```python
from build123d import *

# Parameters (mm, degrees)
ESQUISSE1_R        = 5.5
BOSS_EXTRU_1_DEPTH = 5
ESQUISSE2_W        = 33
ESQUISSE2_H        = 10
ESQUISSE2_W_2      = 10
ESQUISSE2_H_2      = 24.25
ESQUISSE2_H_3      = 12.75
BOSS_EXTRU_2_DEPTH = 6
D_POUILLE1_ANGLE   = 10
BOSS_EXTRU_3_DEPTH = 10
CHANFREIN1_SIZE    = 5


with BuildPart() as part:
    # Esquisse1 → Boss.-Extru.1 (new body)
    with BuildSketch(Plane.XY):
        Polygon((-22.5, 75.232443508), (22.5, 75.232443508), (70, -9.767556492), (70, -54.767556492), (-70, -54.767556492), (-70, -9.767556492), align=None)
        with Locations((0, 60.232443508)):
            Circle(ESQUISSE1_R, mode=Mode.SUBTRACT)
        with Locations((0, 13.982443508)):
            Circle(ESQUISSE1_R, mode=Mode.SUBTRACT)
        with Locations((0, -32.267556492)):
            Circle(ESQUISSE1_R, mode=Mode.SUBTRACT)
        with Locations((-55, -32.267556492)):
            Circle(ESQUISSE1_R, mode=Mode.SUBTRACT)
        with Locations((55, -32.267556492)):
            Circle(ESQUISSE1_R, mode=Mode.SUBTRACT)
    extrude(amount=BOSS_EXTRU_1_DEPTH)

    # Esquisse2 → Boss.-Extru.2 (add)
    with BuildSketch(Plane.XY.offset(5)):
        with Locations((-27.5, -32.267556492)):
            Rectangle(ESQUISSE2_W, ESQUISSE2_H)
        with Locations((27.5, -32.267556492)):
            Rectangle(ESQUISSE2_W, ESQUISSE2_H)
        with Locations((0, 37.107443508)):
            Rectangle(ESQUISSE2_W_2, ESQUISSE2_H_2)
        with Locations((0, -3.392556492)):
            Rectangle(ESQUISSE2_W_2, ESQUISSE2_H_3)
    extrude(amount=BOSS_EXTRU_2_DEPTH)

    # Dépouille1
    d_pouille1_faces = [part.faces().sort_by_distance(p)[0] for p in [
        (44, -32.267556492, 8),
        (27.5, -27.267556492, 8),
        (-11, -32.267556492, 8),
        (-27.5, -27.267556492, 8),
        (0, 2.982443508, 8),
        (5, -3.392556492, 8),
        (0, 49.232443508, 8),
        (5, 37.107443508, 8),
        (-5, 37.107443508, 8),
        (0, 24.982443508, 8),
        (11, -32.267556492, 8),
        (-44, -32.267556492, 8),
        (-5, -3.392556492, 8),
        (-27.5, -37.267556492, 8),
        (27.5, -37.267556492, 8),
        (0, -9.767556492, 8),
    ]]
    draft(d_pouille1_faces, Plane.XY.offset(5), D_POUILLE1_ANGLE)

    # Esquisse3 → Boss.-Extru.3 (add)
    with BuildSketch(Plane.XY.offset(5)):
        Polygon((-22.75, 74.785075087), (-22.75, -9.517556492), (-69.860294118, -9.517556492), align=None)
        Polygon((22.75, -9.517556492), (69.860294118, -9.517556492), (22.75, 74.785075087), align=None)
    extrude(amount=BOSS_EXTRU_3_DEPTH)

    # Chanfrein1
    chanfrein1_edges = [part.edges().sort_by_distance(p)[0] for p in [
        (-22.75, -9.517556492, 10),
        (22.75, -9.517556492, 10),
    ]]
    chamfer(chanfrein1_edges, length=CHANFREIN1_SIZE)


solid = part.part
```
The model under review builds one solid part; all positions refer to its coordinate system, in mm. A direction names the side the tool comes from. Round coordinates to 2 decimals unless told otherwise and drop trailing zeros. Loops run counter-clockwise (first coordinate to the right, second up) from the corner with the lowest first, then second, coordinate; pieces in that order, holes last.
Item 1: Take a section at A-A (z = 12.75). Write out the cut boundary in (x, y), then the cut area to 3 significant figures.
Determined:
outline: (-69.86, -9.52) - (-27.75, -9.52) - (-22.75, -4.52) - (-22.75, 74.79) - close; (22.75, -4.52) - (27.75, -9.52) - (69.86, -9.52) - (22.75, 74.79) - close
area: 3,950 mm2
Item 2: Take a section at B-B (x = 0). Write out the cut boundary in (y, z).
Determined:
outline: (-54.77, 0) - (-37.77, 0) - (-37.77, 5) - (-54.77, 5) - close; (-26.77, 0) - (8.48, 0) - (8.48, 5) - (2.98, 5) - (1.92, 11) - (-8.71, 11) - (-9.77, 5) - (-26.77, 5) - close; (19.48, 0) - (54.73, 0) - (54.73, 5) - (49.23, 5) - (48.17, 11) - (26.04, 11) - (24.98, 5) - (19.48, 5) - close; (65.73, 0) - (75.23, 0) - (75.23, 5) - (65.73, 5) - close
Item 3: Take a section at C-C (x = -16). Write out the cut boundary in (y, z), then the cut area to 3 significant figures.
Determined:
outline: (-54.77, 0) - (75.23, 0) - (75.23, 5) - (-27.27, 5) - (-28.33, 11) - (-36.21, 11) - (-37.27, 5) - (-54.77, 5) - close
area: 704 mm2
Item 4: For line 1 (Y direction, x = 0, z = 3); line 2 (X direction, y = -28.5, z = 3); line 3 (X direction, y = -31, z = 1.75), list the stretches that pass through material, from the lowest coordinate up.
Determined:
line 1: y = -54.77 to -37.77, -26.77 to 8.48, 19.48 to 54.73, 65.73 to 75.23
line 2: x = -70 to -59.01, -50.99 to -4.01, 4.01 to 50.99, 59.01 to 70
line 3: x = -70 to -60.35, -49.65 to -5.35, 5.35 to 49.65, 60.35 to 70
Item 5: For faces 4 (the face through (27.27, -27.79, 7.96)), 5 (the face through (22.75, 36, 10)), 6 (the face through (27, -32, 11)), list the 3-axis set-ups (+Z, -Z, +X, -X, +Y, -Y) from which the entire face can be reached by the end or side of a thin tool; tool diameter is ignored.
Determined:
face 4: +Z, +X, -X
face 5: +Z, +Y
face 6: +Z, +X, -X, -Y
Item 6: Clearance check with flat-ended pins moving along their axes: pin 1 Ø8.5 at (x, y) = (0.5, -2.5) entering from +Z; pin 2 Ø3 at (y, z) = (41, 10) entering from +X; pin 3 Ø4 at (y, z) = (47.5, 8.5) entering from -X. State where each tip first meets the part, or that it passes through.
Determined:
pin 1: stops at z = 11
pin 2: stops at x = 42.47
pin 3: stops at x = -39.12
Item 7: Take a section at D-D (x = 55). Write out the cut boundary in (y, z).
Determined:
outline: (-54.77, 0) - (-37.77, 0) - (-37.77, 5) - (-54.77, 5) - close; (-26.77, 0) - (17.07, 0) - (17.07, 15) - (-9.52, 15) - (-9.52, 5) - (-26.77, 5) - close
Item 8: Mouldability with a two-part tool opening along X and no side actions: class faces 1 (the face through (4.48, -3.48, 7.96)), 2 (the face through (70, -32, 2)), 3 (the face through (-49, -9.518, 10)) as released by +X, released by -X, zero draft, split by the parting line, or undercut.
Determined:
face 1: undercut
face 2: released by +X
face 3: zero draft
